Part model, mm, in its own coordinate system. A direction names the side the tool comes from. Give positions to 0.01 mm unless a question says otherwise; leave off trailing zeros. Loops run counter-clockwise (first coordinate to the right, second up) from the corner with the lowest first, then second, coordinate; pieces in that order, holes last. Notation, with made-up numbers: (-27, -40) -> (20, -40) arc R29 ccw to (20, -16) -> close; hole circle Ø11 at (1.25, 44). An arc over 180 degrees is marked (long way). Write item = value, one per line.
from build123d import *

# Parameters (mm, degrees)
SKETCH1_R                = 73
BOSS_EXTRUDE1_DEPTH      = 12.5
SKETCH1_3_R              = 76
SKETCH1_3_R_2            = 73
BOSS_EXTRUDE2_DEPTH      = 10
BOSS_EXTRUDE3_DEPTH      = 32.5
BOSS_EXTRUDE3_DEPTH_BACK = 12.5
FILLET1_R                = 3


with BuildPart() as part:
    # Sketch1 → Boss-Extrude1 (new, symmetric)
    with BuildSketch(Plane(origin=(0, 0, 0), x_dir=(1, 0, 0), z_dir=(0, 1, 0))):
        with Locations(Location((0, 0, 0), (0, 0, 270))):
            Circle(SKETCH1_R)
        with BuildLine():
            ThreePointArc((-13, 49.477267507), (-14.234954784, 51.903090128), (-16.923076923, 52.331725248))
            ThreePointArc((-16.923076923, 52.331725248), (-44.473414703, 32.359162298), (-55, 0))
            ThreePointArc((-55, 0), (-52.788696317, -2.770263795), (-49.597249509, -1.227897839))
            ThreePointArc((-49.597249509, -1.227897839), (-35.501955289, 17.007275211), (-15.172413793, 27.865847763))
            ThreePointArc((-15.172413793, 27.865847763), (-13.603882451, 28.944274456), (-13, 30.749439459))
            Line((-13, 30.749439459), (-13, 49.477267507))
        make_face(mode=Mode.SUBTRACT)
        with BuildLine():
            ThreePointArc((16.923076923, 52.331725248), (14.234954784, 51.903090128), (13, 49.477267507))
            Line((13, 49.477267507), (13, 30.749439459))
            ThreePointArc((13, 30.749439459), (13.603882451, 28.944274456), (15.172413793, 27.865847763))
            ThreePointArc((15.172413793, 27.865847763), (35.501955289, 17.007275211), (49.597249509, -1.227897839))
            ThreePointArc((49.597249509, -1.227897839), (52.788696317, -2.770263795), (55, 0))
            ThreePointArc((55, 0), (44.473414703, 32.359162298), (16.923076923, 52.331725248))
        make_face(mode=Mode.SUBTRACT)
        with BuildLine():
            ThreePointArc((23.467803367, 7.392317069), (17.76019792, 15.978270251), (8, 19.3))
            Line((8, 19.3), (-8, 19.3))
            ThreePointArc((-8, 19.3), (-17.76019792, 15.978270251), (-23.467803367, 7.392317069))
            ThreePointArc((-23.467803367, 7.392317069), (0, -65), (23.467803367, 7.392317069))
        make_face(mode=Mode.SUBTRACT)
    extrude(amount=BOSS_EXTRUDE1_DEPTH, both=True)

    # Sketch1_3 → Boss-Extrude2 (add, symmetric)
    with BuildSketch(Plane(origin=(0, 0, 0), x_dir=(1, 0, 0), z_dir=(0, 1, 0))):
        with Locations(Location((0, 0, 0), (0, 0, 270))):
            Circle(SKETCH1_3_R)
        with Locations(Location((0, 0, 0), (0, 0, 270))):
            Circle(SKETCH1_3_R_2, mode=Mode.SUBTRACT)
    extrude(amount=BOSS_EXTRUDE2_DEPTH, both=True)

    # Sketch1_4 → Boss-Extrude3 (add, two sides: drawn at the far end of the back side and taken through both)
    with BuildSketch(Plane(origin=(0, 0, 0), x_dir=(1, 0, 0), z_dir=(0, 1, 0)).offset(-BOSS_EXTRUDE3_DEPTH_BACK)):
        with BuildLine():
            ThreePointArc((-23.467803367, 7.392317069), (0, -65), (23.467803367, 7.392317069))
            ThreePointArc((23.467803367, 7.392317069), (17.76019792, 15.978270251), (8, 19.3))
            Line((8, 19.3), (-8, 19.3))
            ThreePointArc((-8, 19.3), (-17.76019792, 15.978270251), (-23.467803367, 7.392317069))
        make_face()
        with BuildLine():
            ThreePointArc((-8, -1.314561435), (0, -50), (8, -1.314561435))
            Line((8, -1.314561435), (8, 4.3))
            Line((8, 4.3), (-8, 4.3))
            Line((-8, 4.3), (-8, -1.314561435))
        make_face(mode=Mode.SUBTRACT)
    extrude(amount=BOSS_EXTRUDE3_DEPTH + BOSS_EXTRUDE3_DEPTH_BACK)

    # Fillet1
    fillet1_edges = [part.edges().sort_by_distance(p)[0] for p in [
        (-23.467803367, 22.5, -7.392317069),
        (23.467803367, 22.5, -7.392317069),
        (0, 32.5, -19.3),
        (-17.76019792, 32.5, -15.978270251),
        (0, 32.5, 65),
        (17.76019792, 32.5, -15.978270251),
        (17.76019792, 12.5, -15.978270251),
        (0, 12.5, 65),
        (-17.76019792, 12.5, -15.978270251),
        (0, 12.5, -19.3),
    ]]
    fillet(fillet1_edges, radius=FILLET1_R)


solid = part.part
1) Drop flat-ended pins along their axis: P1, Ø12, axis at y = 15.5, z = -52.5, coming from the +X side; P2, Ø15.5, axis at x = 0.5, y = 22.5, coming from the -Z side; P3, Ø1, axis at x = 60.5, y = 14.5, coming from the -Z side; P4, Ø4.5, axis at y = 2, z = -1.5, coming from the -X side. Give the stop position or say it passes through.
Resolved:
P1 = 57.15
P2 = -19.4
P3 = through
P4 = -76
2) Which spindle directions (+Z, -Z, +X, -X, +Y, -Y) get a long thin tool onto all of the face, cutting with end or side? Do faces 1 (the face through (-71.264, -11.232, -15.825)), 2 (the face through (-1.394, 22.402, 64.976)), 3 (the face through (17.506, 22.402, -16.17)), 4 (the face through (-25, 32.5, 22)), 5 (the face through (8, 10, -1)). Say none if no direction does.
Resolved:
face_1 = -Y
face_2 = +Y
face_3 = -Z, +X, +Y
face_4 = +Z, -Z, +X, -X, +Y
face_5 = +Y, -Y
3) Pull direction X, two halves, no side cores. Call faces 6 (the face through (29, 10, -68)), 7 (the face through (-46.245, 0.14, -60.311)), 8 (the face through (-52.84, 0.18, 2.76)), 9 (the face through (52.74, 0.18, 2.78)): pulls with the +X half, pulls with the -X half, needs draft (parallel to the pull), parting line crosses it, or undercut.
Resolved:
face_6 = needs draft
face_7 = parting line crosses it
face_8 = undercut
face_9 = undercut
4) Slice it at A-A, the plane y = -8. List the corners of the cut face in (x, z), and give its area (3 significant figures).
Resolved:
outline = circle Ø152 at (0, 0); hole (-55, 0) arc R55 ccw to (-16.92, -52.33) arc R3 ccw to (-13, -49.48) -> (-13, -30.75) arc R3 ccw to (-15.17, -27.87) arc R55 cw to (-49.6, 1.23) arc R2.84 ccw to start; hole (-8, -4.3) -> (8, -4.3) -> (8, 1.31) arc R25 ccw (long way) to (-8, 1.31) -> close; hole (13, -49.48) arc R3 ccw to (16.92, -52.33) arc R55 ccw to (55, 0) arc R2.84 ccw to (49.6, 1.23) arc R55 cw to (15.17, -27.87) arc R3 ccw to (13, -30.75) -> close
area = 14,100 mm²
5) Drill centre lines: line 1 along X through (y, z) = (26.5, 25.5) (3 decimals); line 2 along Y through (x, z) = (39, 1); line 3 along X through (y, z) = (4.5, -30). Where is each one in solid material? Low to high. Write a range as [from, to].
Resolved:
line_1 = [-39.997, -24.995], [24.995, 39.997]
line_2 = [-12.5, 12.5]
line_3 = [-69.83, -46.1], [-13.1, 13.1], [46.1, 69.83]
